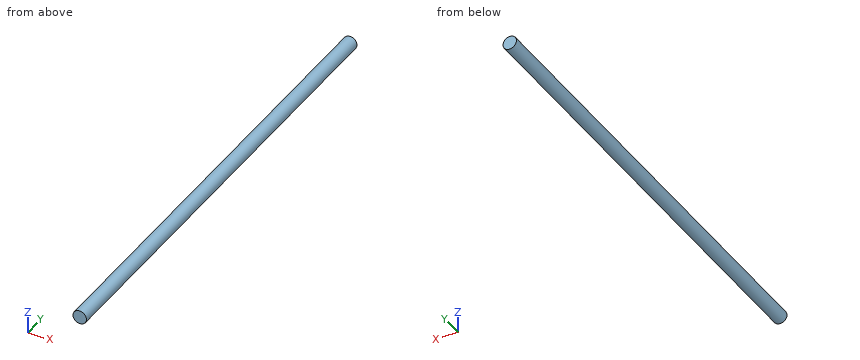
from build123d import *

# Parameters (mm, degrees)
F0_R     = 4
F1_DEPTH = 400
F2_DEPTH = 100
F3_DEPTH = 25


with BuildPart() as f1:
    # F0 (on Front) → F1 (new body)
    with BuildSketch(Plane.XZ):
        Circle(F0_R)
    extrude(amount=F1_DEPTH)

    # F2 (cut): a face of the model
    f2_faces = [f1.faces().sort_by_distance(p)[0] for p in [
        (0, -400, 0),
    ]]
    extrude(f2_faces, amount=-F2_DEPTH, mode=Mode.SUBTRACT)

    # F3 (cut): a face of the model
    f3_faces = [f1.faces().sort_by_distance(p)[0] for p in [
        (0, -300, 0),
    ]]
    extrude(f3_faces, amount=-F3_DEPTH, mode=Mode.SUBTRACT)


solid = f1.part
CAD build for the part. Positions are in the model's coordinates, mm. Round coordinates to 2 decimals unless told otherwise and drop trailing zeros. Write each loop counter-clockwise with the first axis right and the second up, starting at its lowest first coordinate (ties: lowest second). Pieces come first, ordered by that corner, then holes. Notation, with made-up numbers: M 31.5,86 L 49.5,86 A18 ccw 49.5,114 Z; hole C 0,73.25 d9. An arc over 180 degrees is marked long. Use a Markdown table: item, result. Add a question column.
1. Drill centre lines: probe 1 along X at (y, z) = (-238, 0.25); probe 2 along X at (y, z) = (-92, -3). Where is each one in solid material? Low to high.
2. Flat gauge pin, fed straight in: P1, Ø2, axis at x = -1, z = -1.5, coming from the +Y side. Where does the tip first touch, or does it go through?
3. Slice it at C-C on x = 1.75. Give the cut face in (y, z).
4. Slice it at B-B on y = -174. Give the cut face in (x, z).
5. Slice it at A-A on z = 1.5. Give the cut face in (x, y).
Reply:
| question | item | result |
|---|---|---|
| 1 | probe 1 | x = -3.99 to 3.99 |
| 1 | probe 2 | x = -2.65 to 2.65 |
| 2 | P1 | stops at y = 0 |
| 3 | outline | M -275,-3.6 L 0,-3.6 L 0,3.6 L -275,3.6 Z |
| 4 | outline | C 0,0 d8 |
| 5 | outline | M -3.71,-275 L 3.71,-275 L 3.71,0 L -3.71,0 Z |
